Work out the finished part from the listing and answer in its coordinate system (mm). A direction names the side the tool comes from. Coordinates: 2 decimals unless noted, no trailing zeros. Order: outer loops, then holes, each group sorted by start corner. A loop starts at its lowest first (then second) coordinate and runs counter-clockwise, first axis right, second up. Notation, with made-up numbers: (-33.75, 48.25) - (10.25, 48.25) arc R29 ccw to (10.25, 83.25) - close; hole circle Ø6 at (84.25, 32). An arc over 180 degrees is marked (long way). Answer as a JSON object with one key per item and string values. Group by question number.
1) Section C-C (y = 40) is taken. Give the vertices of the cut face in (x, z).
2) The mould has two halves that part along X. Classify faces 3 (the face through (-40, 5, 5)), 4 (the face through (-1, -27, 167)), 5 (the face through (97.25, -1, 82)): released by +X, released by -X, zero draft, split by the parting line, or undercut.
3) Each of these flat-tipped pins is pushed along its axis until it touches: P1, Ø7, axis at x = 42.5, y = 8, coming from the +Z side; P2, Ø5, axis at x = 42.25, y = 7, coming from the +Z side; P3, Ø4, axis at x = 69, y = 56, coming from the +Z side; P4, Ø12, axis at x = 63, z = 87.5, coming from the +Y side. Where does it stop, or does it pass through?
4) Find the intervals of material crossed by line 1 along Y through (x, z) = (42, 70); line 2 along Y through (x, z) = (-42.25, 2.7); line 3 along X through (y, z) = (4, 64.5), in increasing order.
5) Section D-D (z = 144) is taken. Give the vertices of the cut face in (x, y), plus the area to 3 significant figures.
6) Section B-B (x = -13.5) is taken. Give the vertices of the cut face in (y, z).
7) A tool of negligible diameter and unlimited length cuts with its end or side. For faces 1 (the face through (-40, 7, 2)), 2 (the face through (-43.18, 2.8, 87.13)), from which of +Z, -Z, +X, -X, +Y, -Y can it reach the whole face along a straight path? Write none if from no direction.
8) Section A-A (z = 92) is taken. Give the vertices of the cut face in (x, y), plus the area to 3 significant figures.
from build123d import *

# Parameters (mm, degrees)
SKIZZE2_W                                           = 194.5
SKIZZE2_H                                           = 144
AUFSATZ_LINEAR_AUSTRAGEN1_DEPTH                     = 167
STIRNSENKUNG_F_R_M4_SENKSCHRAUBE_KOPF_B_D           = 4.5
STIRNSENKUNG_F_R_M4_SENKSCHRAUBE_KOPF_B_CBORE_D     = 8.6
STIRNSENKUNG_F_R_M4_SENKSCHRAUBE_KOPF_B_CBORE_DEPTH = 162
SCHNITT_LINEAR_AUSTRAGEN1_DEPTH                     = 267.27664186


with BuildPart() as part:
    # Skizze2 → Aufsatz-Linear austragen1 (new body)
    with BuildSketch(Plane.XY):
        Rectangle(SKIZZE2_W, SKIZZE2_H)
    extrude(amount=AUFSATZ_LINEAR_AUSTRAGEN1_DEPTH)

    # Stirnsenkung für M4 Senkschraube (Kopf Button)1 (through all)
    with Locations(Plane.XY.offset(167)):
        with Locations((-42.25, 7)):
            stirnsenkung_f_r_m4_senkschraube_kopf_b = CounterBoreHole(STIRNSENKUNG_F_R_M4_SENKSCHRAUBE_KOPF_B_D / 2, STIRNSENKUNG_F_R_M4_SENKSCHRAUBE_KOPF_B_CBORE_D / 2, STIRNSENKUNG_F_R_M4_SENKSCHRAUBE_KOPF_B_CBORE_DEPTH)

    # Spiegeln1: Stirnsenkung für M4 Senkschraube (Kopf Button)1 across plane
    add(stirnsenkung_f_r_m4_senkschraube_kopf_b.mirror(Plane(origin=(0, 0, 0), x_dir=(0, 0, 1), z_dir=(1, 0, 0))), mode=Mode.SUBTRACT)

    # Skizze6 → Schnitt-Linear austragen1 (cut, through all)
    with BuildSketch(Plane.ZY.offset(97.25)):
        Polygon((70.87118018, 72), (167, 16.5), (205.188147907, 84.754255682), (82.593849392, 116.819294381), align=None)
    extrude(amount=-SCHNITT_LINEAR_AUSTRAGEN1_DEPTH, mode=Mode.SUBTRACT)


solid = part.part
Report:
{
 "1": {"outline": "(-97.25, 0) - (97.25, 0) - (97.25, 126.3) - (-97.25, 126.3) - close"},
 "2": {"face 3": "undercut", "face 4": "zero draft", "face 5": "released by +X"},
 "3": {"P1": "stops at z = 167", "P2": "stops at z = 5", "P3": "stops at z = 102.05", "P4": "stops at y = 65.86"},
 "4": {"line 1": "y = -72 to 2.71, 11.29 to 72", "line 2": "y = -72 to 4.75, 9.25 to 72", "line 3": "x = -97.25 to -45.33, -39.17 to 39.17, 45.33 to 97.25"},
 "5": {"outline": "(-97.25, -72) - (97.25, -72) - (97.25, 29.78) - (-97.25, 29.78) - close; hole circle Ø8.6 at (-42.25, 7); hole circle Ø8.6 at (42.25, 7)", "area": "19,700 mm²"},
 "6": {"outline": "(-72, 0) - (72, 0) - (72, 70.87) - (16.5, 167) - (-72, 167) - close"},
 "7": {"face 1": "+Z, -Z", "face 2": "+Z"},
 "8": {"outline": "(-97.25, -72) - (97.25, -72) - (97.25, 59.8) - (-97.25, 59.8) - close; hole circle Ø8.6 at (-42.25, 7); hole circle Ø8.6 at (42.25, 7)", "area": "25,500 mm²"}
}
